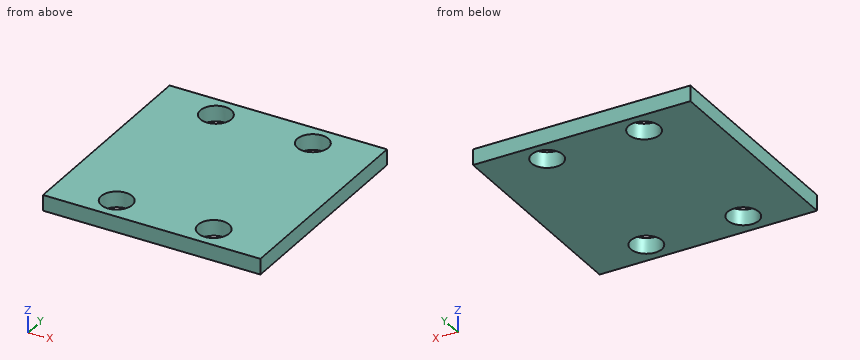
from build123d import *

# Parameters (mm, degrees)
SKETCH1_W             = 22.858863977
SKETCH1_H             = 22.839779742
BOSS_EXTRUDE1_DEPTH   = 0.825
F_4_CLEARANCE_HOLE1_D = 3.2639


with BuildPart() as part:
    # Sketch1 → Boss-Extrude1 (new, symmetric)
    with BuildSketch(Plane.XY):
        with Locations((11.429431989, 11.419889871)):
            Rectangle(SKETCH1_W, SKETCH1_H)
    extrude(amount=BOSS_EXTRUDE1_DEPTH, both=True)

    # #4 Clearance Hole1 (through all)
    with Locations(Plane.XY.offset(0.825)):
        with Locations((16.483506518, 20.400756331), (6.289658732, 20.400756331), (6.289658732, 2.503280726), (16.483506518, 2.503280726)):
            Hole(F_4_CLEARANCE_HOLE1_D / 2)


solid = part.part
Build history of the part. All positions in model axes, mm. Round coordinates to 2 decimals unless told otherwise and drop trailing zeros. Write each loop counter-clockwise with the first axis right and the second up, starting at its lowest first coordinate (ties: lowest second). Pieces come first, ordered by that corner, then holes. Notation, with made-up numbers: M -40,1 L -17,1 A31 cw -17,29 Z; hole C -3,-2 d11. An arc over 180 degrees is marked long. Answer in a Markdown table with one row per item.
1. Saw through at B-B (z = -0.1). List the corners of the cut face in (x, y), and give its area (3 significant figures).
Geometry check:
| item | result |
|---|---|
| outline | M 0,0 L 22.86,0 L 22.86,22.84 L 0,22.84 Z; hole C 6.29,2.5 d3.26; hole C 6.29,20.4 d3.26; hole C 16.48,2.5 d3.26; hole C 16.48,20.4 d3.26 |
| area | 489 mm2 |
2. Saw through at A-A (x = 17.25). List the corners of the cut face in (y, z) (1 decimal), and give its area (3 significant figures).
Geometry check:
| item | result |
|---|---|
| outline | M 0,-0.8 L 1.1,-0.8 L 1.1,0.8 L 0,0.8 Z; M 3.9,-0.8 L 19,-0.8 L 19,0.8 L 3.9,0.8 Z; M 21.8,-0.8 L 22.8,-0.8 L 22.8,0.8 L 21.8,0.8 Z |
| area | 28.2 mm2 |
3. Probe L1, parallel to Y at x = 16, z = -0.2; L2, parallel to Y at x = 15.5, z = -0.2; L3, parallel to X at y = 21.25, z = 0.3. List the from-to ranges inside material, lowest first. Write a range as [from, to].
Geometry check:
| item | result |
|---|---|
| L1 | [0, 0.94], [4.06, 18.84], [21.96, 22.84] |
| L2 | [0, 1.2], [3.81, 19.1], [21.7, 22.84] |
| L3 | [0, 4.9], [7.68, 15.09], [17.88, 22.86] |
4. Flat gauge pins, fed straight in: P1, Ø2, axis at x = 6.29, y = 2.5, coming from the -Z side; P2, Ø4, axis at x = 16.48, y = 2.5, coming from the +Z side (3 decimals). Where does each tip first touch, or does it go through?
Geometry check:
| item | result |
|---|---|
| P1 | through |
| P2 | z = 0.825 |
5. Saw through at C-C (x = 7.5). List the corners of the cut face in (y, z) (3 decimals).
Geometry check:
| item | result |
|---|---|
| outline | M 0,-0.825 L 1.409,-0.825 L 1.409,0.825 L 0,0.825 Z; M 3.598,-0.825 L 19.306,-0.825 L 19.306,0.825 L 3.598,0.825 Z; M 21.495,-0.825 L 22.84,-0.825 L 22.84,0.825 L 21.495,0.825 Z |
